Job drawing, mm, ordinate dimensions from the low corner. One solid piece. Round coordinates to 2 decimals unless told otherwise and drop trailing zeros. Loops run counter-clockwise (first coordinate to the right, second up) from the corner with the lowest first, then second, coordinate; pieces in that order, holes last. Notation, with made-up numbers: M -36.5,34 L -26.5,34 A24 cw -26.5,49 Z; hole C 2,66 d3. An arc over 180 degrees is marked long. Put each result on its own line as item: value. Start each with the question number.
1) Slice it at B-B on z = 20. Give the cut face in (x, y).
2) Probe line 1 along X through (y, z) = (0.9, 23.5); line 2 along X through (y, z) = (0.35, 17); line 3 along Z through (x, y) = (11, 1.6). List the from-to ranges inside material, lowest first.
3) Slice it at D-D on x = 7.5. Give the cut face in (y, z), then the cut area to 3 significant figures.
4) Slice it at A-A on y = 1.4. Give the cut face in (x, z).
5) Drop flat-ended pins along their axis: pin 1 Ø1 at (x, y) = (8.5, 1) entering from +Z; pin 2 Ø1 at (x, y) = (13, 1.5) entering from +Z; pin 3 Ø0.6 at (x, y) = (5, 1) entering from -Z. Give the stop position or say it passes through.
6) Slice it at C-C on x = 25. Give the cut face in (y, z).
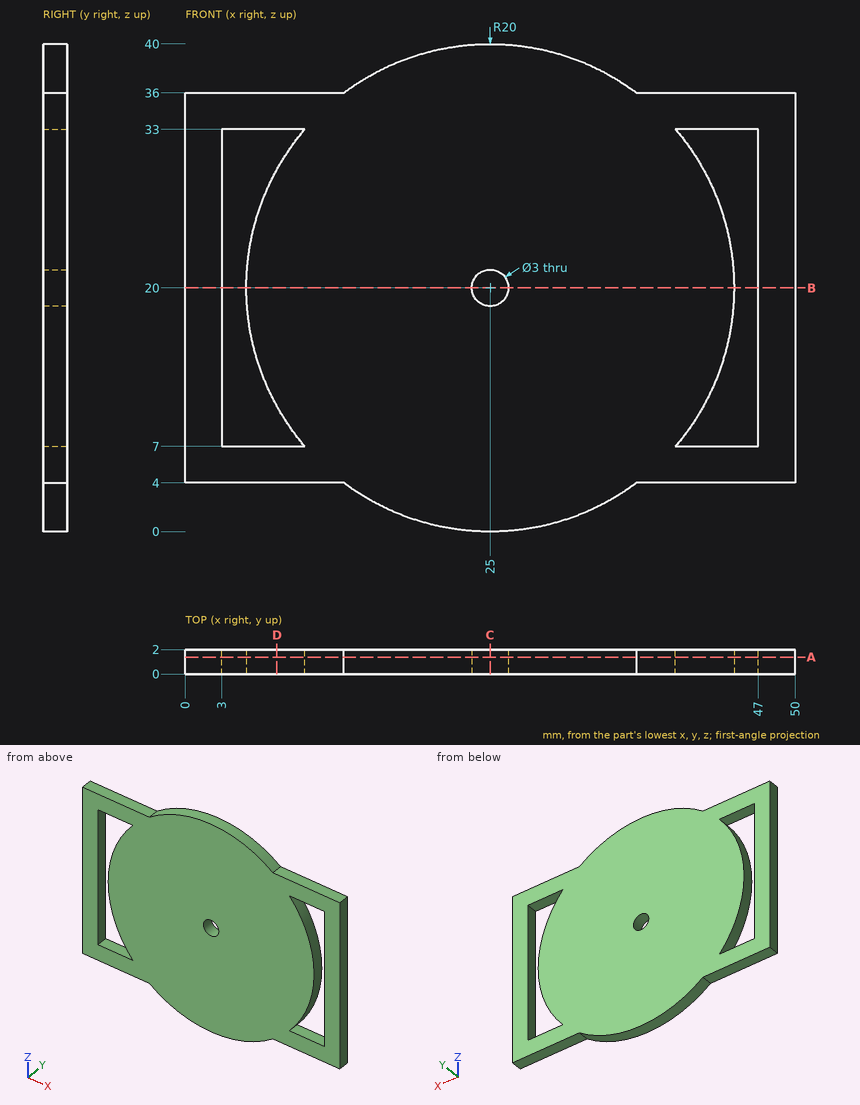
Recorded:
1. outline: M 0,0 L 3,0 L 3,2 L 0,2 Z; M 5,0 L 23.5,0 L 23.5,2 L 5,2 Z; M 26.5,0 L 45,0 L 45,2 L 26.5,2 Z; M 47,0 L 50,0 L 50,2 L 47,2 Z
2. line 1: x = 0 to 3, 5.31 to 44.69, 47 to 50
2. line 2: x = 0 to 3, 5.23 to 44.77, 47 to 50
2. line 3: z = 4 to 36
3. outline: M 0,4 L 2,4 L 2,7 L 0,7 Z; M 0,10.32 L 2,10.32 L 2,29.68 L 0,29.68 Z; M 0,33 L 2,33 L 2,36 L 0,36 Z
3. area: 50.7 mm2
4. outline: M 0,4 L 13,4 A20 ccw 37,4 L 50,4 L 50,36 L 37,36 A20 ccw 13,36 L 0,36 Z; hole M 3,7 L 9.8,7 A20 cw 9.8,33 L 3,33 Z; hole C 25,20 d3; hole M 40.2,7 L 47,7 L 47,33 L 40.2,33 A20 cw Z
5. pin 1: stops at z = 36
5. pin 2: stops at z = 36.36
5. pin 3: stops at z = 4
6. outline: M 0,0 L 2,0 L 2,18.5 L 0,18.5 Z; M 0,21.5 L 2,21.5 L 2,40 L 0,40 Z
